Read the model definition and answer for the solid it produces. Units are mm, in the model's axes. A direction names the side the tool comes from. Round coordinates to 2 decimals unless told otherwise and drop trailing zeros. Order: outer loops, then holes, each group sorted by start corner. A loop starts at its lowest first (then second) coordinate and runs counter-clockwise, first axis right, second up. Notation, with made-up numbers: (-39, 87.5) -> (-14, 87.5) arc R16 cw to (-14, 115.5) -> close; hole circle Ø8 at (52.25, 21.25). An arc over 180 degrees is marked (long way). One line per item, written item: value. Start each with the question number.
1. Section C-C (y = -16) is taken. Give the vertices of the cut face in (x, z) (3 decimals), then the cut area to 3 significant figures.
2. Section A-A (x = -7.25) is taken. Give the vertices of the cut face in (y, z) (3 decimals), then the cut area to 3 significant figures.
3. Section B-B (z = -7.75) is taken. Give the vertices of the cut face in (x, y) (3 decimals), then the cut area to 3 significant figures.
4. Section D-D (z = 0) is taken. Give the vertices of the cut face in (x, y) (3 decimals), then the cut area to 3 significant figures.
5. A flat-ended cylindrical pin translates along its axis: pin 1 Ø4 at (y, z) = (-12.7, 0) entering from +X. Find the tip coordinate at first contact, or state that the pin passes through.
6. The mould has two halves that part along Y. Classify faces 3 (the face through (0, 0, 9.525)), 4 (the face through (11, 25.4, 0)), 5 (the face through (11.13, -10.6, -1.34)): released by +Y, released by -Y, zero draft, split by the parting line, or undercut.
7. For faces 1 (the face through (9.525, 0, 0)), 2 (the face through (11.13, 15.17, 0.32)), determine the directions among +Z, -Z, +X, -X, +Y, -Y from which every point of the face is accessible in a straight line to the end or side of a thin tool.
8. Consider line 1 (Y direction, x = 11.15, z = 0); line 2 (Z direction, x = -4.25, y = -19) (3 decimals). Determine where each line is inside the solid, lowest interval first.
from build123d import *

# Parameters (mm, degrees)
SKETCH1_W           = 25.4
SKETCH1_H           = 25.4
SKETCH1_W_2         = 19.05
SKETCH1_H_2         = 19.05
EXTRUDE_THIN1_DEPTH = 25.4
SKETCH2_R           = 2.4892
CUT_EXTRUDE1_DEPTH  = 26.4


with BuildPart() as part:
    # Sketch1 → Extrude-Thin1 (new body, symmetric)
    with BuildSketch(Plane(origin=(0, 0, 0), x_dir=(1, 0, 0), z_dir=(0, 1, 0))):
        Rectangle(SKETCH1_W, SKETCH1_H)
        Rectangle(SKETCH1_W_2, SKETCH1_H_2, mode=Mode.SUBTRACT)
    extrude(amount=EXTRUDE_THIN1_DEPTH, both=True)

    # Sketch2 → Cut-Extrude1 (cut, through all)
    with BuildSketch(Plane(origin=(12.7, 0, 0), x_dir=(0, 0, -1), z_dir=(1, 0, 0))):
        with Locations((0, 12.7)):
            Circle(SKETCH2_R)
        with Locations((0, -12.7)):
            Circle(SKETCH2_R)
    extrude(amount=-CUT_EXTRUDE1_DEPTH, mode=Mode.SUBTRACT)


solid = part.part
Answer:
1. outline: (-12.7, -12.7) -> (12.7, -12.7) -> (12.7, 12.7) -> (-12.7, 12.7) -> close; hole (-9.525, -9.525) -> (9.525, -9.525) -> (9.525, 9.525) -> (-9.525, 9.525) -> close
1. area: 282 mm^2
2. outline: (-25.4, -12.7) -> (25.4, -12.7) -> (25.4, -9.525) -> (-25.4, -9.525) -> close; (-25.4, 9.525) -> (25.4, 9.525) -> (25.4, 12.7) -> (-25.4, 12.7) -> close
2. area: 323 mm^2
3. outline: (-12.7, -25.4) -> (-9.525, -25.4) -> (-9.525, 25.4) -> (-12.7, 25.4) -> close; (9.525, -25.4) -> (12.7, -25.4) -> (12.7, 25.4) -> (9.525, 25.4) -> close
3. area: 323 mm^2
4. outline: (-12.7, -25.4) -> (-9.525, -25.4) -> (-9.525, -15.189) -> (-12.7, -15.189) -> close; (-12.7, -10.211) -> (-9.525, -10.211) -> (-9.525, 10.211) -> (-12.7, 10.211) -> close; (-12.7, 15.189) -> (-9.525, 15.189) -> (-9.525, 25.4) -> (-12.7, 25.4) -> close; (9.525, -25.4) -> (12.7, -25.4) -> (12.7, -15.189) -> (9.525, -15.189) -> close; (9.525, -10.211) -> (12.7, -10.211) -> (12.7, 10.211) -> (9.525, 10.211) -> close; (9.525, 15.189) -> (12.7, 15.189) -> (12.7, 25.4) -> (9.525, 25.4) -> close
4. area: 259 mm^2
5. pin 1: through
6. face 3: zero draft
6. face 4: released by +Y
6. face 5: undercut
7. face 1: +Y, -Y
7. face 2: +X, -X
8. line 1: -25.4 to -15.19, -10.21 to 10.21, 15.19 to 25.4
8. line 2: -12.7 to -9.525, 9.525 to 12.7
